Verification items for the finished model (mm, model axes). A direction names the side the tool comes from. Coordinates: 2 decimals unless noted, no trailing zeros. Write each loop counter-clockwise with the first axis right and the second up, starting at its lowest first coordinate (ties: lowest second). Pieces come first, ordered by that corner, then holes. Notation, with made-up numbers: (55, 35) -> (67, 35) arc R32 cw to (67, 64) -> close; hole circle Ø8 at (46.5, 13). An arc over 180 degrees is marked (long way). Write item = value, one per line. Start each with the question number.
(1) Section check B-B (y = 25.4). Record the cut outline in (x, z).
(2) Section check A-A (x = 0). Record the cut outline in (y, z), plus the area to 3 significant figures.
(3) Section check C-C (y = 0). Record the cut outline in (x, z).
(4) Section check D-D (x = 113.03). Record the cut outline in (y, z).
(5) Mould release check, pull along Y, two halves, no side actions. Record for faces 4 (the face through (108.03, -5, 5)), 5 (the face through (113, -30.4, 5)), 6 (the face through (-1.825, -1.4, 4.93)): released by +Y, released by -Y, zero draft, split by the parting line, or undercut.
(6) Gauge pin test, flat ends, axial feed: pin 1 Ø3.5 at (x, y) = (113.03, 0) entering from -Z; pin 2 Ø5 at (y, z) = (-6, 6) entering from -X; pin 3 Ø5 at (x, z) = (95.5, 5.5) entering from -Y. Record the tip position at first contact, or that the pin passes through.
(7) Material ranges on probe 1 along Y at (x, z) = (113.03, 5.5); probe 2 along X at (y, z) = (9, 7); probe 3 along X at (y, z) = (-0.5, 1) (3 decimals), recorded low to high. Write a range as [from, to].
(8) Set-up check for faces 1 (the face through (0, -5, 5)), 2 (the face through (-5, 13, 5)), 3 (the face through (56, 20.4, 5)): record each of +Z, -Z, +X, -X, +Y, -Y from which the full face is reachable in a straight line by a thin tool's end or side.
```python
from build123d import *

# Parameters (mm, degrees)
SKETCH1_R           = 2.3
BOSS_EXTRUDE1_DEPTH = 10


with BuildPart() as part:
    # Sketch1 → Boss-Extrude1 (new body)
    with BuildSketch(Plane.XY):
        Polygon((108.03, -30.4), (118.03, -30.4), (118.03, 30.4), (-5, 30.4), (-5, -5), (5, -5), (5, 20.4), (108.03, 20.4), align=None)
        Circle(SKETCH1_R, mode=Mode.SUBTRACT)
        with Locations((113.03, 0)):
            Circle(SKETCH1_R, mode=Mode.SUBTRACT)
        with Locations((113.03, -25.4)):
            Circle(SKETCH1_R, mode=Mode.SUBTRACT)
        with Locations((113.03, 25.4)):
            Circle(SKETCH1_R, mode=Mode.SUBTRACT)
    extrude(amount=BOSS_EXTRUDE1_DEPTH)


solid = part.part
```
Response:
q1.outline = (-5, 0) -> (110.73, 0) -> (110.73, 10) -> (-5, 10) -> close; (115.33, 0) -> (118.03, 0) -> (118.03, 10) -> (115.33, 10) -> close
q2.outline = (-5, 0) -> (-2.3, 0) -> (-2.3, 10) -> (-5, 10) -> close; (2.3, 0) -> (30.4, 0) -> (30.4, 10) -> (2.3, 10) -> close
q2.area = 308 mm2
q3.outline = (-5, 0) -> (-2.3, 0) -> (-2.3, 10) -> (-5, 10) -> close; (2.3, 0) -> (5, 0) -> (5, 10) -> (2.3, 10) -> close; (108.03, 0) -> (110.73, 0) -> (110.73, 10) -> (108.03, 10) -> close; (115.33, 0) -> (118.03, 0) -> (118.03, 10) -> (115.33, 10) -> close
q4.outline = (-30.4, 0) -> (-27.7, 0) -> (-27.7, 10) -> (-30.4, 10) -> close; (-23.1, 0) -> (-2.3, 0) -> (-2.3, 10) -> (-23.1, 10) -> close; (2.3, 0) -> (23.1, 0) -> (23.1, 10) -> (2.3, 10) -> close; (27.7, 0) -> (30.4, 0) -> (30.4, 10) -> (27.7, 10) -> close
q5.face_4 = zero draft
q5.face_5 = released by -Y
q5.face_6 = undercut
q6.pin_1 = through
q6.pin_2 = -5
q6.pin_3 = 20.4
q7.probe_1 = [-30.4, -27.7], [-23.1, -2.3], [2.3, 23.1], [27.7, 30.4]
q7.probe_2 = [-5, 5], [108.03, 118.03]
q7.probe_3 = [-5, -2.245], [2.245, 5], [108.03, 110.785], [115.275, 118.03]
q8.face_1 = +Z, -Z, -X, -Y
q8.face_2 = +Z, -Z, -X, +Y, -Y
q8.face_3 = +Z, -Z, -Y
